from build123d import *

# Parameters (mm, degrees)
BOSS_EXTRUDE1_DEPTH = 5.5
SHELL1_T            = -0.254


with BuildPart() as part:
    # Sketch1 → Boss-Extrude1 (new body)
    with BuildSketch(Plane.XY):
        Polygon((-2.7, 0), (2.7, 0), (3.9, 1.35), (3.9, 2.45), (-3.9, 2.45), (-3.9, 1.35), align=None)
    extrude(amount=BOSS_EXTRUDE1_DEPTH)

    # Shell1
    shell1_openings = [part.faces().sort_by_distance(p)[0] for p in [
        (0, 1.266666667, 5.5),
    ]]
    offset(amount=SHELL1_T, openings=shell1_openings, kind=Kind.INTERSECTION)


solid = part.part
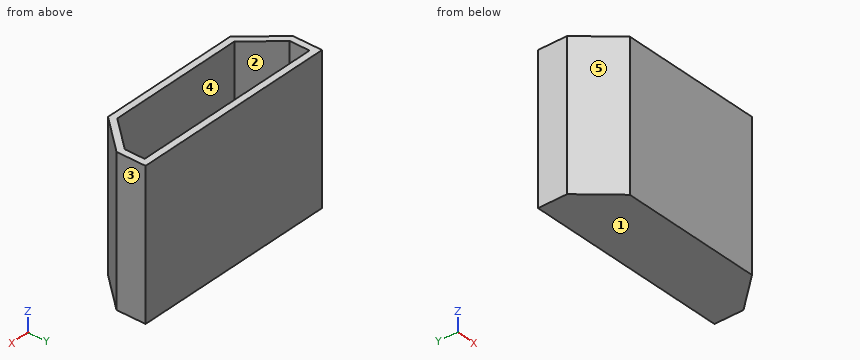
Work out the finished part from the listing and answer in its coordinate system (mm). Face numbers are marked on the shaded views. A direction names the side the tool comes from. Coordinates: 2 decimals unless noted, no trailing zeros. Loops run counter-clockwise (first coordinate to the right, second up) from the corner with the lowest first, then second, coordinate; pieces in that order, holes last. Notation, with made-up numbers: (31, 16.25) -> (74, 16.25) arc R19 ccw to (74, 51.25) -> close; hole circle Ø2 at (10, 31). An arc over 180 degrees is marked (long way). Write each question's results on one line, items separated by ' | '. Start each with the question number.
1) Find section C-C on y = 1.6. Determine the outline of the cut face in (x, z), then the cut area to 3 significant figures.
2) Find section B-B on x = -1.75. Determine the outline of the cut face in (y, z).
3) The mould has two halves that part along X. Classify the marked faces 1, 2 and 3: pulls with the +X half, pulls with the -X half, needs draft (parallel to the pull), parting line crosses it, or undercut.
4) For the marked faces 4 and 5, determine the directions among +Z, -Z, +X, -X, +Y, -Y from which every point of the face is accessible in a straight line to the end or side of a thin tool.
5) Consider line 1 along Y through (x, z) = (-0.5, 2.8); line 2 along X through (y, z) = (1.8, 5.1); line 3 along Z through (x, y) = (3, 0.85). Determine where each line is inside the solid, lowest interval first.
6) Find section A-A on z = 2.95. Determine the outline of the cut face in (x, y), then the cut area to 3 significant figures.
Response values:
1) outline: (-3.9, 0) -> (3.9, 0) -> (3.9, 5.5) -> (3.65, 5.5) -> (3.65, 0.25) -> (-3.65, 0.25) -> (-3.65, 5.5) -> (-3.9, 5.5) -> close | area: 4.65 mm^2
2) outline: (0, 0) -> (2.45, 0) -> (2.45, 5.5) -> (2.2, 5.5) -> (2.2, 0.25) -> (0.25, 0.25) -> (0.25, 5.5) -> (0, 5.5) -> close
3) face 1: needs draft | face 2: undercut | face 3: pulls with the +X half
4) face 4: +Z | face 5: +Z, -Z, -X, -Y
5) line 1: y = 0 to 0.25, 2.2 to 2.45 | line 2: x = -3.9 to -3.65, 3.65 to 3.9 | line 3: z = 0 to 0.25
6) outline: (-3.9, 1.35) -> (-2.7, 0) -> (2.7, 0) -> (3.9, 1.35) -> (3.9, 2.45) -> (-3.9, 2.45) -> close; hole (-3.65, 1.45) -> (-2.59, 0.25) -> (2.59, 0.25) -> (3.65, 1.45) -> (3.65, 2.2) -> (-3.65, 2.2) -> close | area: 4.59 mm^2
